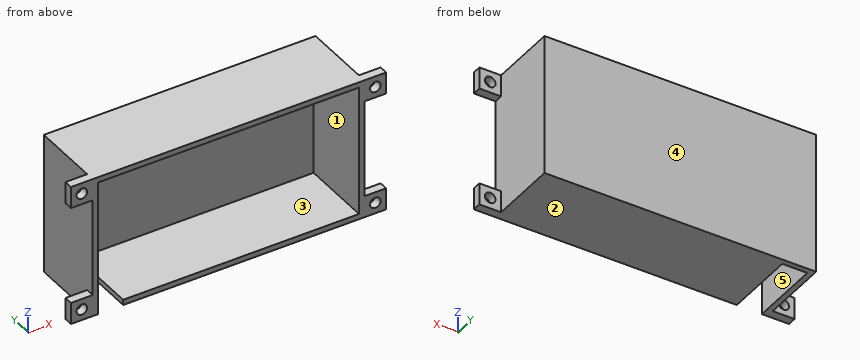
from build123d import *

# Parameters (mm, degrees)
SKETCH1_W           = 79.375
SKETCH1_H           = 41.275
SKETCH1_W_2         = 76.2
SKETCH1_H_2         = 38.1
BOSS_EXTRUDE1_DEPTH = 20.955
SKETCH2_W           = 79.375
SKETCH2_H           = 41.275
BOSS_EXTRUDE2_DEPTH = 1.5875
SKETCH3_W           = 6.35
SKETCH3_H           = 6.35
SKETCH3_R           = 1.55
BOSS_EXTRUDE3_DEPTH = 2.54
SKETCH4_W           = 8.89
SKETCH4_H           = 1.5875
CUT_EXTRUDE1_DEPTH  = 20.955
BOSS_EXTRUDE4_REACH = 97.72
SKETCH5_W           = 1.5875
SKETCH5_H           = 1.5875


with BuildPart() as part:
    # Sketch1 → Boss-Extrude1 (new body)
    with BuildSketch(Plane(origin=(0, 0, 0), x_dir=(1, 0, 0), z_dir=(0, 1, 0))):
        with Locations((38.1, 19.05)):
            Rectangle(SKETCH1_W, SKETCH1_H)
        with Locations((38.1, 19.05)):
            Rectangle(SKETCH1_W_2, SKETCH1_H_2, mode=Mode.SUBTRACT)
    extrude(amount=BOSS_EXTRUDE1_DEPTH)

    # Sketch2 → Boss-Extrude2 (add)
    with BuildSketch(Plane(origin=(0, 20.955, 0), x_dir=(1, 0, 0), z_dir=(0, 1, 0))):
        with Locations((38.1, 19.05)):
            Rectangle(SKETCH2_W, SKETCH2_H)
    extrude(amount=BOSS_EXTRUDE2_DEPTH)

    # Sketch3 → Boss-Extrude3 (add)
    # profile 1 of 4: a face of its own
    with BuildSketch(Plane.XZ):
        with Locations((80.9625, -36.5125)):
            Rectangle(SKETCH3_W, SKETCH3_H)
        with Locations(Location((80.9625, -36.5125, 0), (0, 0, 270))):
            Circle(SKETCH3_R, mode=Mode.SUBTRACT)
    # profile 2 of 4: a face of its own
    with BuildSketch(Plane.XZ):
        with Locations((80.9625, -1.5875)):
            Rectangle(SKETCH3_W, SKETCH3_H)
        with Locations(Location((80.9625, -1.5875, 0), (0, 0, 90))):
            Circle(SKETCH3_R, mode=Mode.SUBTRACT)
    # profile 3 of 4: a face of its own
    with BuildSketch(Plane.XZ):
        with Locations((-4.7625, -1.5875)):
            Rectangle(SKETCH3_W, SKETCH3_H)
        with Locations(Location((-4.7625, -1.5875, 0), (0, 0, 270))):
            Circle(SKETCH3_R, mode=Mode.SUBTRACT)
    # profile 4 of 4: a face of its own
    with BuildSketch(Plane.XZ):
        with Locations((-4.7625, -36.5125)):
            Rectangle(SKETCH3_W, SKETCH3_H)
        with Locations(Location((-4.7625, -36.5125, 0), (0, 0, 90))):
            Circle(SKETCH3_R, mode=Mode.SUBTRACT)
    extrude(amount=-BOSS_EXTRUDE3_DEPTH)

    # Sketch4 → Cut-Extrude1 (cut)
    with BuildSketch(Plane.XZ):
        with Locations((2.8575, -38.89375)):
            Rectangle(SKETCH4_W, SKETCH4_H)
    extrude(amount=-CUT_EXTRUDE1_DEPTH, mode=Mode.SUBTRACT)

    # Sketch5 → Boss-Extrude4 (add, up to next)
    with BuildSketch(Plane.XZ, mode=Mode.PRIVATE) as boss_extrude4_sk1:
        with Locations((-0.79375, -38.89375)):
            Rectangle(SKETCH5_W, SKETCH5_H)
    boss_extrude4_tool1 = extrude(boss_extrude4_sk1.sketch, amount=-BOSS_EXTRUDE4_REACH, mode=Mode.PRIVATE) - part.part
    add(boss_extrude4_tool1.solids().sort_by_distance((-0.79375, 0, -38.89375))[0])


solid = part.part
Input: part model. Units: mm. Frame: model coordinates. Face numbers are marked on the shaded views. A direction names the side the tool comes from. Round coordinates to 2 decimals unless told otherwise and drop trailing zeros. Write each loop counter-clockwise with the first axis right and the second up, starting at its lowest first coordinate (ties: lowest second). Pieces come first, ordered by that corner, then holes.
1) Cut plane B-B (x = 62.5). Return the cut outline in (y, z) (1 decimal).
2) Draft query along X for the marked faces 1 and 2. Return one class per face: pulls with the +X half, pulls with the -X half, needs draft (parallel to the pull), parting line crosses it, or undercut.
3) Cut plane C-C (z = -18.5). Return the cut outline in (x, y) (1 decimal).
4) Ray query, L1, parallel to Z at x = 53.5, y = 17; L2, parallel to X at y = 2.25, z = -27; L3, parallel to Z at x = 3.5, y = 12.5. Return the intervals inside material, ascending.
5) Cut plane A-A (y = 8). Return the cut outline in (x, z).
6) Contact query for flat-ended pins moving along their axis: P1, Ø6.5, axis at y = 5.5, z = -25, coming from the -X side; P2, Ø4, axis at x = 80.96, z = -1.59, coming from the +Y side; P3, Ø8, axis at y = 9, z = -3, coming from the +X side. Output: stop coordinate, or through.
7) Reachability of the marked faces 3, 4 and 5 from +Z, -Z, +X, -X, +Y, -Y: full face, straight path, thin tool, end or side. Return the list, or none.
Geometry says:
1. outline: (0, -39.7) - (22.5, -39.7) - (22.5, 1.6) - (0, 1.6) - (0, 0) - (21, 0) - (21, -38.1) - (0, -38.1) - close
2. face 1: undercut
2. face 2: needs draft
3. outline: (-1.6, 0) - (0, 0) - (0, 21) - (76.2, 21) - (76.2, 0) - (77.8, 0) - (77.8, 22.5) - (-1.6, 22.5) - close
4. L1: z = -39.69 to -38.1, 0 to 1.59
4. L2: x = -1.59 to 0, 76.2 to 77.79
4. L3: z = 0 to 1.59
5. outline: (-1.59, -39.69) - (0, -39.69) - (0, 0) - (76.2, 0) - (76.2, -38.1) - (7.3, -38.1) - (7.3, -39.69) - (77.79, -39.69) - (77.79, 1.59) - (-1.59, 1.59) - close
6. P1: stops at x = -1.59
6. P2: stops at y = 2.54
6. P3: stops at x = 77.79
7. face 3: -Y
7. face 4: +Z, -Z, +X, -X, +Y
7. face 5: -Z, -Y
